The listing builds one solid part. Answer for the finished solid, in the listing's coordinates (mm). A direction names the side the tool comes from. Round coordinates to 2 decimals unless told otherwise and drop trailing zeros. Loops run counter-clockwise (first coordinate to the right, second up) from the corner with the lowest first, then second, coordinate; pieces in that order, holes last. Notation, with made-up numbers: (-21, 11) -> (8, 11) arc R23 cw to (8, 22) -> close; hole circle Ø2 at (-21.5, 53). An arc over 180 degrees is marked (long way). Answer in a Markdown table with one row per item. Add a question column.
```python
from build123d import *

# Parameters (mm, degrees)
F0_R     = 18.49
F1_DEPTH = 80.85
F2_R     = 1.5
F2_R_2   = 6.5
F3_DEPTH = 9.6


with BuildPart() as f1:
    # F0 (on Top) → F1 (new body)
    with BuildSketch(Plane.XY):
        Circle(F0_R)
    extrude(amount=F1_DEPTH)

    # F2 (on face) → F3 (cut)
    with BuildSketch(Plane.XY.offset(80.85)):
        with Locations((10.407604, -11.74129)):
            Circle(F2_R)
        with Locations((15.372057, 3.142604)):
            Circle(F2_R)
        with Locations((4.964453, 14.883894)):
            Circle(F2_R)
        with Locations((-10.407604, 11.74129)):
            Circle(F2_R)
        with Locations((-15.372057, -3.142604)):
            Circle(F2_R)
        with Locations((-4.964453, -14.883894)):
            Circle(F2_R)
        with Locations((1.602135, -7.836848)):
            Circle(F2_R_2)
    extrude(amount=-F3_DEPTH, mode=Mode.SUBTRACT)


solid = f1.part
```
Item 1: Section D-D, the plane x = 0 is taken. Write down the section's boundary in (y, z), and give its area (3 significant figures).
Item 2: Section A-A, the plane x = -15 is taken. Write down the section's boundary in (y, z).
Item 3: Section C-C, the plane y = 7 is taken. Write down the section's boundary in (x, z).
Item 4: Section B-B, the plane z = 59.5 is taken. Write down the section's boundary in (x, y).
Item 5: The mould has two halves that part along X. Classify faces 3 (the cylindrical face through (-13.94, -2.69, 76.12)), 4 (the flat face through (0, 0, 0)), 5 (the cylindrical face through (-4.01, -18.05, 39.86)): +X half, -X half, draft (parallel to the pull), parting line (faces both ways), or undercut.
Item 6: For faces 1 (the flat face through (0, 0, 80.85)), 2 (the flat face through (-15, -3, 71.25)), determine the directions among +Z, -Z, +X, -X, +Y, -Y from which every point of the face is accessible in a straight line to the end or side of a thin tool.
Item 7: Flat-ended cylindrical pins translate along their axes: P1, Ø2.5, axis at x = 10.41, y = -11.74, coming from the +Z side; P2, Ø5, axis at y = -12, z = 17.5, coming from the +X side; P3, Ø1.5, axis at y = 1, z = 52, coming from the +X side. Find the tip coordinate at first contact, or state that the pin passes through.
Item 8: Consider L1, parallel to Z at x = 6.5, y = -8.5; L2, parallel to Y at x = -3.5, z = 63.5; L3, parallel to Y at x = -4.5, z = 41. Determine where each line is inside the solid, lowest interval first. Write a range as from..to.
Here are the results:
| question | item | result |
|---|---|---|
| 1 | outline | (-18.49, 0) -> (18.49, 0) -> (18.49, 80.85) -> (-1.54, 80.85) -> (-1.54, 71.25) -> (-14.14, 71.25) -> (-14.14, 80.85) -> (-18.49, 80.85) -> close |
| 1 | area | 2,870 mm² |
| 2 | outline | (-10.81, 0) -> (10.81, 0) -> (10.81, 80.85) -> (-1.69, 80.85) -> (-1.69, 71.25) -> (-4.6, 71.25) -> (-4.6, 80.85) -> (-10.81, 80.85) -> close |
| 3 | outline | (-17.11, 0) -> (17.11, 0) -> (17.11, 80.85) -> (-17.11, 80.85) -> close |
| 4 | outline | circle Ø36.98 at (0, 0) |
| 5 | face 3 | undercut |
| 5 | face 4 | draft |
| 5 | face 5 | parting line |
| 6 | face 1 | +Z, +X, -X, +Y, -Y |
| 6 | face 2 | +Z |
| 7 | P1 | stops at z = 71.25 |
| 7 | P2 | stops at x = 15.86 |
| 7 | P3 | stops at x = 18.49 |
| 8 | L1 | z = 0..71.25 |
| 8 | L2 | y = -18.16..18.16 |
| 8 | L3 | y = -17.93..17.93 |
